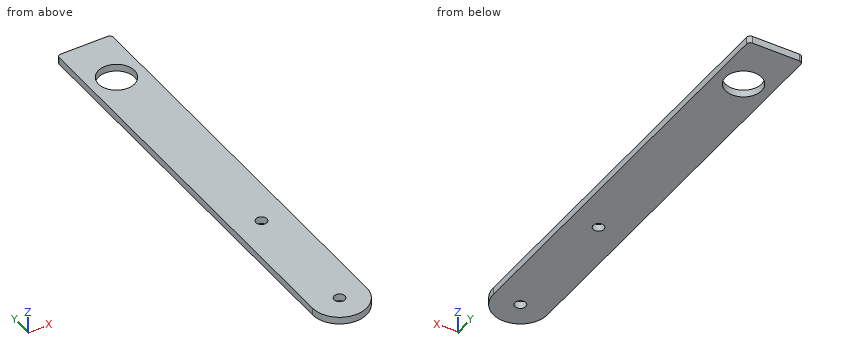
from build123d import *

# Parameters (mm, degrees)
SKETCH2_R           = 1.5
SKETCH2_R_2         = 5
BOSS_EXTRUDE2_DEPTH = 2
SKETCH3_R           = 1.5
CUT_EXTRUDE1_DEPTH  = 2
FILLET1_R           = 1


with BuildPart() as part:
    # Sketch2 → Boss-Extrude2 (new body)
    with BuildSketch(Plane.XY):
        with BuildLine():
            Line((0, 6.5), (0, 100))
            Line((0, 100), (0, 121))
            Line((0, 121), (7.5, 121))
            Line((7.5, 121), (15, 121))
            Line((15, 121), (15, 100))
            Line((15, 100), (15, 6.5))
            ThreePointArc((15, 6.5), (7.5, -1), (0, 6.5))
        make_face()
        with Locations((7.5, 6.5)):
            Circle(SKETCH2_R, mode=Mode.SUBTRACT)
        with Locations((7.5, 106.5)):
            Circle(SKETCH2_R_2, mode=Mode.SUBTRACT)
    extrude(amount=BOSS_EXTRUDE2_DEPTH)

    # Sketch3 → Cut-Extrude1 (cut)
    with BuildSketch(Plane.XY.offset(2)):
        with Locations((7.5, 41.5)):
            Circle(SKETCH3_R)
    extrude(amount=-CUT_EXTRUDE1_DEPTH, mode=Mode.SUBTRACT)

    # Fillet1
    fillet1_edges = [part.edges().sort_by_distance(p)[0] for p in [
        (0, 121, 1),
        (15, 121, 1),
    ]]
    fillet(fillet1_edges, radius=FILLET1_R)


solid = part.part
Design review of the part built by this model. Coordinates are the model's own, in mm. Coordinates: 2 decimals unless noted, no trailing zeros. Order: outer loops, then holes, each group sorted by start corner. A loop starts at its lowest first (then second) coordinate and runs counter-clockwise, first axis right, second up.
Item 1: For line 1 (Y direction, x = 7.5, z = 0.6); line 2 (Y direction, x = 6.75, z = 0.55); line 3 (Y direction, x = 11.5, z = 0.9), list the stretches that pass through material, from the lowest coordinate up.
Item 2: Take a section at D-D, the plane y = 41.5. Write out the cut boundary in (x, z), then the cut area to 3 significant figures.
Item 3: Take a section at B-B, the plane x = 7.5. Write out the cut boundary in (y, z), then the cut area to 3 significant figures.
Item 4: Take a section at C-C, the plane z = 0.35. Write out the cut boundary in (x, y), then the cut area to 3 significant figures.
Item 5: Take a section at A-A, the plane y = 106.5. Write out the cut boundary in (x, z).
The answers:
1. line 1: y = -1 to 5, 8 to 40, 43 to 101.5, 111.5 to 121
1. line 2: y = -0.96 to 5.2, 7.8 to 40.2, 42.8 to 101.56, 111.44 to 121
1. line 3: y = 0.16 to 103.5, 109.5 to 121
2. outline: (0, 0) - (6, 0) - (6, 2) - (0, 2) - close; (9, 0) - (15, 0) - (15, 2) - (9, 2) - close
2. area: 24.0 mm2
3. outline: (-1, 0) - (5, 0) - (5, 2) - (-1, 2) - close; (8, 0) - (40, 0) - (40, 2) - (8, 2) - close; (43, 0) - (101.5, 0) - (101.5, 2) - (43, 2) - close; (111.5, 0) - (121, 0) - (121, 2) - (111.5, 2) - close
3. area: 212 mm2
4. outline: (0, 6.5) arc R7.5 ccw to (15, 6.5) - (15, 120) arc R1 ccw to (14, 121) - (1, 121) arc R1 ccw to (0, 120) - close; hole circle Ø10 at (7.5, 106.5); hole circle Ø3 at (7.5, 6.5); hole circle Ø3 at (7.5, 41.5)
4. area: 1,710 mm2
5. outline: (0, 0) - (2.5, 0) - (2.5, 2) - (0, 2) - close; (12.5, 0) - (15, 0) - (15, 2) - (12.5, 2) - close
